Study the drawing (mm; zero at the part's minimum x, y, z) and answer. Coordinates: 2 decimals unless noted, no trailing zeros. Loops run counter-clockwise (first coordinate to the right, second up) from the corner with the lowest first, then second, coordinate; pieces in that order, holes last. Notation, with made-up numbers: (65, 19) - (70, 19) arc R4 ccw to (70, 26) - close; hole circle Ø2 at (89.5, -0.75). An arc over 180 degrees is marked (long way). Use one line per item in the form item = value.
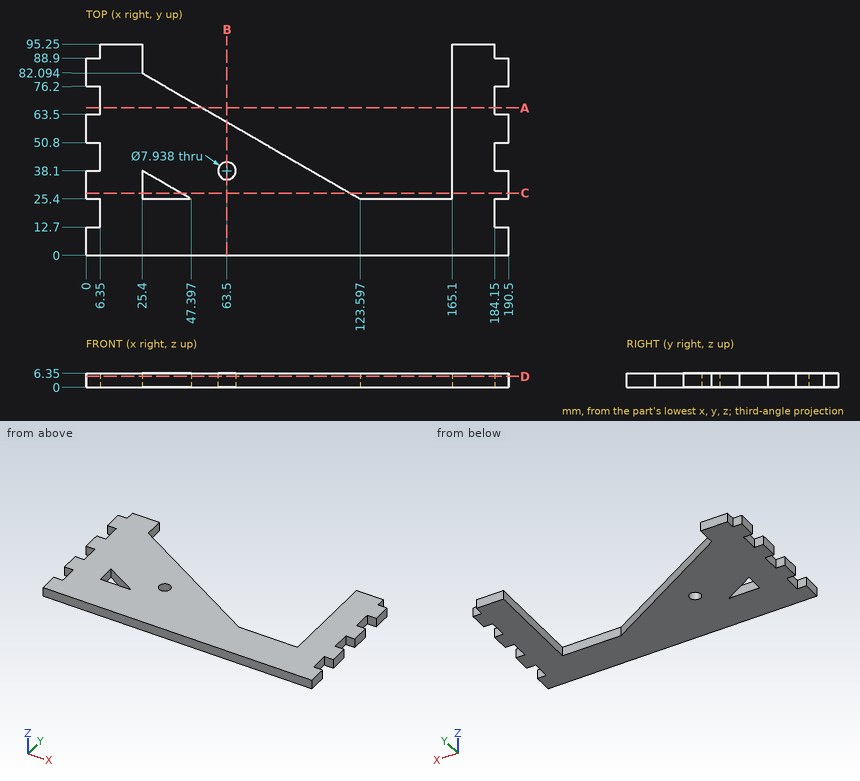
Item 1: The part is cut by section B-B on x = 63.5. Give the vertices of the cut face in (y, z).
Results below:
outline = (0, 0) - (34.13, 0) - (34.13, 6.35) - (0, 6.35) - close; (42.07, 0) - (60.1, 0) - (60.1, 6.35) - (42.07, 6.35) - close
Item 2: The part is cut by section C-C on y = 28. Give the vertices of the cut face in (x, z).
Results below:
outline = (0, 0) - (25.4, 0) - (25.4, 6.35) - (0, 6.35) - close; (42.89, 0) - (119.09, 0) - (119.09, 6.35) - (42.89, 6.35) - close; (165.1, 0) - (190.5, 0) - (190.5, 6.35) - (165.1, 6.35) - close
Item 3: Find the intervals of material crossed by L1, parallel to Y at x = 63.5, z = 3.5 (1 decimal); L2, parallel to X at y = 57.5, z = 1.25 (1 decimal); L3, parallel to X at y = 23.5, z = 5.75, in increasing order.
Results below:
L1 = 0 to 34.1, 42.1 to 60.1
L2 = 0 to 68, 165.1 to 190.5
L3 = 6.35 to 184.15
Item 4: The part is cut by section A-A on y = 66.5. Give the vertices of the cut face in (x, z).
Results below:
outline = (6.35, 0) - (52.41, 0) - (52.41, 6.35) - (6.35, 6.35) - close; (165.1, 0) - (184.15, 0) - (184.15, 6.35) - (165.1, 6.35) - close
Item 5: Each of these flat-tipped pins is pushed along its axis until it touches: P1, Ø3, axis at x = 2, z = 3.5, coming from the +Y side; P2, Ø3, axis at y = 93.5, z = 3, coming from the +X side. Where does it stop, or does it pass through?
Results below:
P1 = 88.9
P2 = 184.15
Item 6: The part is cut by section D-D on z = 5. Count the separate pieces of the cut face and the enclosed holes in it, plus the area to 3 significant figures.
Results below:
separate_pieces = 1
enclosed_holes = 2
area = 10,400 mm²
